Geometry check sheet. Reference: the model listing, model coordinates, mm. A direction names the side the tool comes from. Coordinates: 2 decimals unless noted, no trailing zeros. Write each loop counter-clockwise with the first axis right and the second up, starting at its lowest first coordinate (ties: lowest second). Pieces come first, ordered by that corner, then holes. Notation, with made-up numbers: (46.5, 73.25) -> (58.5, 73.25) arc R35 ccw to (58.5, 112.25) -> close; hole circle Ø4 at (57.5, 50). An arc over 180 degrees is marked (long way). Answer in a Markdown table with one row per item. Add a question column.
1. Cross-section at A-A on z = 4. Record the cut outline in (x, y), and give its area (3 significant figures).
2. Set-up check for faces 4 (the cylindrical face through (-0.54, -2.44, 12.68)), 5 (the flat face through (-7.675, -0.014, 36.989)): record each of +Z, -Z, +X, -X, +Y, -Y from which the full face is reachable in a straight line by a thin tool's end or side.
3. Mould release check, pull along X, two halves, no side actions. Record for faces 1 (the flat face through (1, -1, 0)), 2 (the cylindrical face through (-5.462, 0.751, 38.327)), 3 (the cylindrical face through (0, -1, 13)): pulls with the +X half, pulls with the -X half, needs draft (parallel to the pull), parting line crosses it, or undercut.
4. Scan lines: L1, parallel to Y at x = 0, z = 11; L2, parallel to X at y = 0.4, z = 16; L3, parallel to Z at x = -9.75, y = 0.6. Record each from-to range of solid material in increasing order. Write a range as from..to.
5. Depth check by flat-ended pin: P1, Ø5, axis at x = -1, z = 33, coming from the -Y side; P2, Ø2, axis at y = 1.5, z = 33, coming from the -X side; P3, Ø1.5, axis at y = 1.5, z = 6.5, coming from the +X side. Enter the tip coordinate at first touch or a pass-through.
```python
from build123d import *

# Parameters (mm, degrees)
F1_R = 2.5
F3_R = 2
F5_R = 1


with BuildPart() as f2:
    # F2: sweep along a path in F0
    with BuildLine(Plane.XZ) as f2_path:
        Line((0, 0), (0, 25))
        ThreePointArc((0, 25), (-1.3196601125, 30.5901699437), (-5, 35))
        Line((-5, 35), (-10.3333333333, 39))
    # F1 (on Top) → F2 (sweep)
    with BuildSketch(Plane.XY):
        Circle(F1_R)
    sweep(path=f2_path.line)

    # F3
    f3_edges = [f2.edges().sort_by_distance(p)[0] for p in [
        (-11.833333, 0, 37),
    ]]
    fillet(f3_edges, radius=F3_R)

    # F6: sweep along a path in F4
    with BuildLine(Plane.XZ) as f6_path:
        Line((0, 0), (0, 25))
        ThreePointArc((0, 25), (-1.3196601125, 30.5901699437), (-5, 35))
        Line((-5, 35), (-7.6666666667, 37))
    # F5 (on face) → F6 (sweep, cut)
    with BuildSketch(Plane(origin=(0, 0, 0), x_dir=(1, 0, 0), z_dir=(0, 0, -1))):
        Circle(F5_R)
    sweep(path=f6_path.line, mode=Mode.SUBTRACT)


solid = f2.part
```
Results found:
| question | item | result |
|---|---|---|
| 1 | outline | circle Ø5 at (0, 0); hole circle Ø2 at (0, 0) |
| 1 | area | 16.5 mm^2 |
| 2 | face 4 | -Z |
| 2 | face 5 | none |
| 3 | face 1 | needs draft |
| 3 | face 2 | parting line crosses it |
| 3 | face 3 | undercut |
| 4 | L1 | y = -2.5..-1, 1..2.5 |
| 4 | L2 | x = -2.47..-0.92, 0.92..2.47 |
| 4 | L3 | z = 35.53..39.65 |
| 5 | P1 | stops at y = -2.5 |
| 5 | P2 | stops at x = -7.31 |
| 5 | P3 | stops at x = 2.38 |
